Model file for the job. Use its own axes, mm. Face numbers are marked on the shaded views. A direction names the side the tool comes from. Round coordinates to 2 decimals unless told otherwise and drop trailing zeros. Order: outer loops, then holes, each group sorted by start corner. A loop starts at its lowest first (then second) coordinate and runs counter-clockwise, first axis right, second up. Notation, with made-up numbers: M -16,25 L 7,25 A30 ccw 7,58 Z; hole C 1.5,50 d5. An arc over 180 degrees is marked long. Return JSON: item names as keys, results as strings. Group by question number.
Item 1: Slice it at A-A on z = 10. Write the cut outline in (x, y).
Item 2: Pull direction Z, two halves, no side cores. Call the marked faces 3, 4 and 5: pulls with the +Z half, pulls with the -Z half, needs draft (parallel to the pull), parting line crosses it, or undercut.
Item 3: Which spindle directions (+Z, -Z, +X, -X, +Y, -Y) get a long thin tool onto all of the face, cutting with end or side? Do the marked faces 1 and 2. Say none if no direction does.
Item 4: Probe line 1 along X through (y, z) = (-23, 5.25); line 2 along Z through (x, y) = (-4, 68.5); line 3 along X through (y, z) = (0, 1.55). List the from-to ranges inside material, lowest first.
Item 5: Pin check, flat tip, straight feed: pin 1 Ø5 at (y, z) = (9.43, 10) entering from +X. Stop position of the tip, or through.
Item 6: Slice it at B-B on y = 0. Write the cut outline in (x, z), then the cut area to 3 significant figures.
Item 7: Slice it at D-D on y = 67.5. Write the cut outline in (x, z), then the cut area to 3 significant figures.
Item 8: Slice it at C-C on x = 0. Write the cut outline in (y, z).
from build123d import *

# Parameters (mm, degrees)
SKETCH1_W               = 20
SKETCH1_H               = 159.6
BOSS_EXTRUDE1_DEPTH     = 2
BOSS_EXTRUDE2_DEPTH     = 159.6
CUT_EXTRUDE1_DEPTH      = 83.873638752
CUT_EXTRUDE1_DEPTH_BACK = 83.873638752
SKETCH3_R               = 6.35
CUT_EXTRUDE2_DEPTH      = 85.664278182
CUT_EXTRUDE2_DEPTH_BACK = 85.664278182
SKETCH5_R               = 2.65


with BuildPart() as part:
    # Sketch1 → Boss-Extrude1 (new body)
    with BuildSketch(Plane.XY):
        Rectangle(SKETCH1_W, SKETCH1_H)
    extrude(amount=BOSS_EXTRUDE1_DEPTH)

    # Sketch4 → Boss-Extrude2 (add)
    with BuildSketch(Plane(origin=(0, 79.8, 0), x_dir=(1, 0, 0), z_dir=(0, 1, 0))):
        Polygon((-8, -2), (-10, -2), (-10, -20), (10, -20), (10, -2), (8, -2), (8, -18), (-8, -18), align=None)
    extrude(amount=-BOSS_EXTRUDE2_DEPTH)

    # Sketch3 → Cut-Extrude1 (cut, two sides: drawn at the far end of the back side and taken through both)
    with BuildSketch(Plane(origin=(0, 0, 0), x_dir=(-1, 0, 0), z_dir=(0, 0, -1)).offset(-CUT_EXTRUDE1_DEPTH_BACK)):
        Circle(SKETCH3_R)
    extrude(amount=CUT_EXTRUDE1_DEPTH + CUT_EXTRUDE1_DEPTH_BACK, mode=Mode.SUBTRACT)

    # Sketch5 → Cut-Extrude2 (cut, two sides: drawn at the far end of the back side and taken through both)
    with BuildSketch(Plane(origin=(10, 0, 0), x_dir=(0, 0, -1), z_dir=(1, 0, 0)).offset(-CUT_EXTRUDE2_DEPTH_BACK)):
        with Locations(Location((-10, 50.8, 0), (0, 0, 180))):
            Circle(SKETCH5_R)
        with Locations(Location((-10, 9.434271247, 0), (0, 0, 180))):
            Circle(SKETCH5_R)
    extrude(amount=CUT_EXTRUDE2_DEPTH + CUT_EXTRUDE2_DEPTH_BACK, mode=Mode.SUBTRACT)


solid = part.part
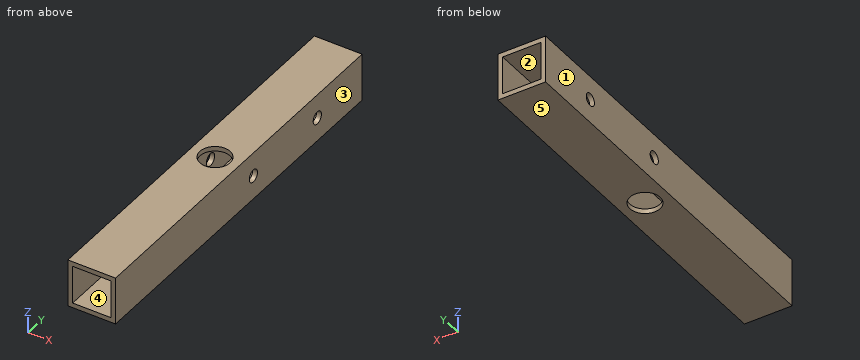
Output values:
{
 "1": {"outline": "M -10,-79.8 L -8,-79.8 L -8,6.78 L -10,6.78 Z; M -10,12.08 L -8,12.08 L -8,48.15 L -10,48.15 Z; M -10,53.45 L -8,53.45 L -8,79.8 L -10,79.8 Z; M 8,-79.8 L 10,-79.8 L 10,6.78 L 8,6.78 Z; M 8,12.08 L 10,12.08 L 10,48.15 L 8,48.15 Z; M 8,53.45 L 10,53.45 L 10,79.8 L 8,79.8 Z"},
 "2": {"face 3": "needs draft", "face 4": "undercut", "face 5": "pulls with the -Z half"},
 "3": {"face 1": "+Z, -Z, -X, +Y, -Y", "face 2": "+Y, -Y"},
 "4": {"line 1": "-10 to -8, 8 to 10", "line 2": "0 to 2, 18 to 20", "line 3": "-10 to -6.35, 6.35 to 10"},
 "5": {"pin 1": "through"},
 "6": {"outline": "M -10,0 L -6.35,0 L -6.35,2 L -8,2 L -8,18 L -6.35,18 L -6.35,20 L -10,20 Z; M 6.35,0 L 10,0 L 10,20 L 6.35,20 L 6.35,18 L 8,18 L 8,2 L 6.35,2 Z", "area": "93.2 mm²"},
 "7": {"outline": "M -10,0 L 10,0 L 10,20 L -10,20 Z; hole M -8,2 L 8,2 L 8,18 L -8,18 Z", "area": "144 mm²"},
 "8": {"outline": "M -79.8,0 L -6.35,0 L -6.35,2 L -79.8,2 Z; M -79.8,18 L -6.35,18 L -6.35,20 L -79.8,20 Z; M 6.35,0 L 79.8,0 L 79.8,2 L 6.35,2 Z; M 6.35,18 L 79.8,18 L 79.8,20 L 6.35,20 Z"}
}
